Here's the drawing with two shaded views (mm, measured from the low corner). I have some questions. A direction names the side the tool comes from. Coordinates: 2 decimals unless noted, no trailing zeros. Write each loop counter-clockwise with the first axis right and the second up, starting at its lowest first coordinate (ties: lowest second). Pieces come first, ordered by that corner, then holes.
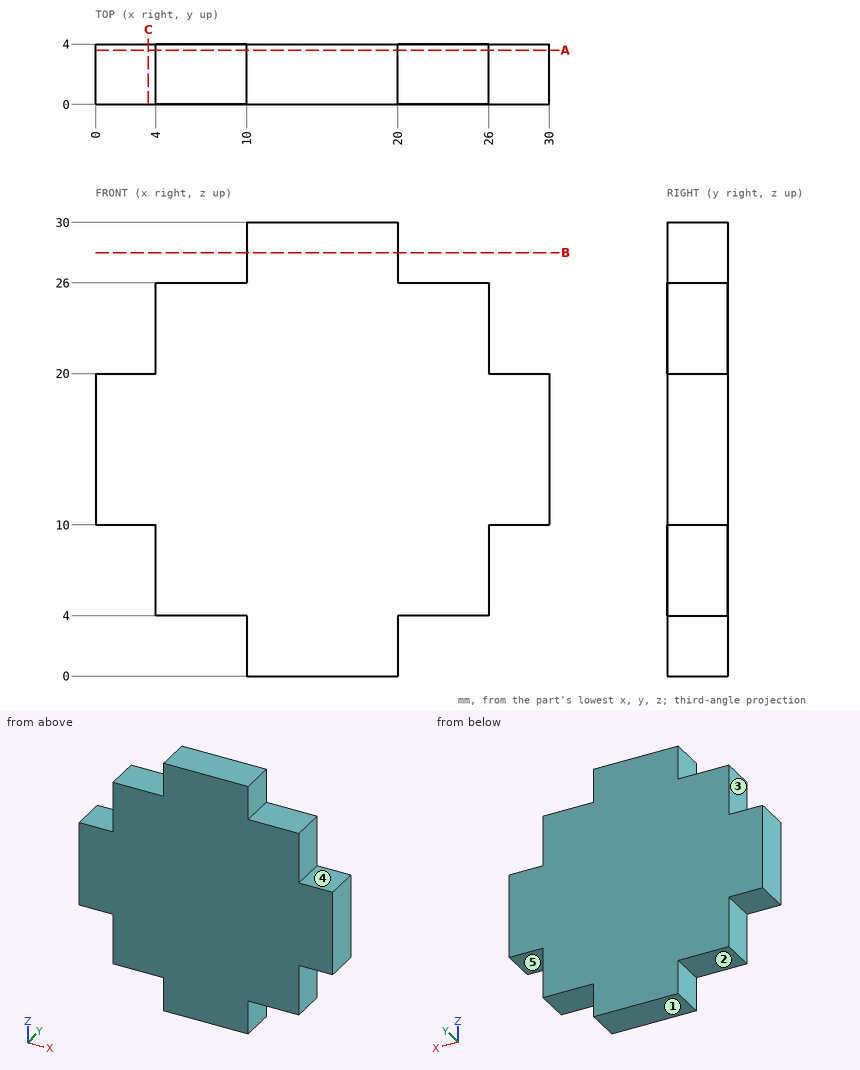
1. I want a section at B-B on z = 28. Please give me the cut outline in (x, y), plus the area to 3 significant figures.
Verdict:
outline: (10, 0) - (20, 0) - (20, 4) - (10, 4) - close
area: 40.0 mm2
2. For pin 1 (2 mm diameter, centred on x = 27.5, y = 2.5, fed in from -Z); pin 2 (1.2 mm diameter, centred on y = 1.5, z = 22.5, fed in from +X); pin 3 (1.2 mm diameter, centred on x = 22, y = 2.5, fed in from -Z), each with a flat end and sliding along its axis, tell me the tip position at first contact or that it passes through.
Verdict:
pin 1: stops at z = 10
pin 2: stops at x = 26
pin 3: stops at z = 4
3. I want a section at C-C on x = 3.5. Please give me the cut outline in (y, z), plus the area to 3 significant figures.
Verdict:
outline: (0, 10) - (4, 10) - (4, 20) - (0, 20) - close
area: 40.0 mm2
4. On a 3-axis mill with a long thin cutter (end or side, diameter ignored), from which of +Z, -Z, +X, -X, +Y, -Y can I reach the whole of each face in a straight line? I mean the marked faces 1, 2, 3, 4 and 5. Say none if no direction works.
Verdict:
face 1: -Z, +X, -X, +Y, -Y
face 2: -Z, -X, +Y, -Y
face 3: +Z, -X, +Y, -Y
face 4: +Z, +X, +Y, -Y
face 5: -Z, +X, +Y, -Y
5. Please list where these lines run through material, in increasing order: line 1 along X through (y, z) = (1.9, 3.75); line 2 along Z through (x, y) = (20.75, 0.95).
Verdict:
line 1: x = 10 to 20
line 2: z = 4 to 26
6. I want a section at A-A on y = 3.6. Please give me the cut outline in (x, z).
Verdict:
outline: (0, 10) - (4, 10) - (4, 4) - (10, 4) - (10, 0) - (20, 0) - (20, 4) - (26, 4) - (26, 10) - (30, 10) - (30, 20) - (26, 20) - (26, 26) - (20, 26) - (20, 30) - (10, 30) - (10, 26) - (4, 26) - (4, 20) - (0, 20) - close
